Can you work these out from the drawing? Everything is in mm from the part's minimum corner. A direction names the side the tool comes from. Coordinates: 2 decimals unless noted, no trailing zeros. Loops run counter-clockwise (first coordinate to the right, second up) from the corner with the lowest first, then second, coordinate; pieces in that order, holes last.
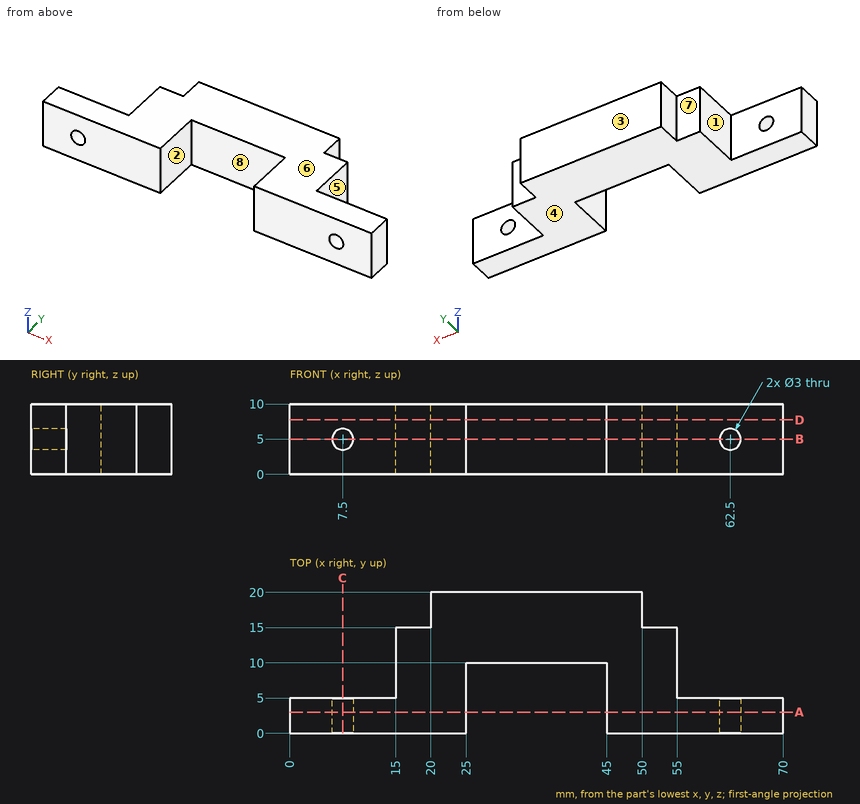
Item 1: I'm going to push flat-ended pins straight in: P1, Ø2, axis at y = 11, z = 3, coming from the +X side; P2, Ø3, axis at x = 63, z = 6.5, coming from the +Y side; P3, Ø2.5, axis at x = 17, z = 6.5, coming from the +Y side. Where does each tip first touch, or does it pass through?
Results are:
P1: stops at x = 55
P2: stops at y = 5
P3: stops at y = 15
Item 2: I need wall thicknesses on line 1 along X through (y, z) = (2.65, 5); line 2 along Z through (x, y) = (62.5, 1.2); line 3 along X through (y, z) = (5.75, 2.75). Which ranges of each line are inside material? Lowest first, please.
Results are:
line 1: x = 0 to 6, 9 to 25, 45 to 61, 64 to 70
line 2: z = 0 to 3.5, 6.5 to 10
line 3: x = 15 to 25, 45 to 55
Item 3: On a 3-axis mill with a long thin cutter (end or side, diameter ignored), from which of +Z, -Z, +X, -X, +Y, -Y can I reach the whole of each face in a straight line? I mean the marked faces 4, 5, 6, 7 and 8. Say none if no direction works.
Results are:
face 4: -Z, +X, -X, +Y, -Y
face 5: +Z, -Z, +X, +Y
face 6: +Z, +X, -X, +Y, -Y
face 7: +Z, -Z, -X, +Y
face 8: +Z, -Z, -Y
Item 4: Suppose I cut it at D-D, the plane z = 7.75. Please give me the cut outline in (x, y), plus the area to 3 significant figures.
Results are:
outline: (0, 0) - (25, 0) - (25, 10) - (45, 10) - (45, 0) - (70, 0) - (70, 5) - (55, 5) - (55, 15) - (50, 15) - (50, 20) - (20, 20) - (20, 15) - (15, 15) - (15, 5) - (0, 5) - close
area: 700 mm2
Item 5: Suppose I cut it at A-A, the plane y = 3. Please give me the cut outline in (x, z), plus the area to 3 significant figures.
Results are:
outline: (0, 0) - (25, 0) - (25, 10) - (0, 10) - close; (45, 0) - (70, 0) - (70, 10) - (45, 10) - close; hole circle Ø3 at (7.5, 5); hole circle Ø3 at (62.5, 5)
area: 486 mm2
Item 6: Suppose I cut it at C-C, the plane x = 7.5. Please give me the cut outline in (y, z).
Results are:
outline: (0, 0) - (5, 0) - (5, 3.5) - (0, 3.5) - close; (0, 6.5) - (5, 6.5) - (5, 10) - (0, 10) - close
Item 7: We'd pull the mould along X, two halves only. Please class the marked faces 1, 2 and 3: +X half, -X half, draft (parallel to the pull), parting line (faces both ways), or undercut.
Results are:
face 1: -X half
face 2: undercut
face 3: draft
Item 8: Suppose I cut it at B-B, the plane z = 5. Please give me the cut outline in (x, y).
Results are:
outline: (0, 0) - (6, 0) - (6, 5) - (0, 5) - close; (9, 0) - (25, 0) - (25, 10) - (45, 10) - (45, 0) - (61, 0) - (61, 5) - (55, 5) - (55, 15) - (50, 15) - (50, 20) - (20, 20) - (20, 15) - (15, 15) - (15, 5) - (9, 5) - close; (64, 0) - (70, 0) - (70, 5) - (64, 5) - close
